The listing builds one solid part. Answer for the finished solid, in the listing's coordinates (mm). Face numbers are marked on the shaded views. A direction names the side the tool comes from. Round coordinates to 2 decimals unless told otherwise and drop trailing zeros. Loops run counter-clockwise (first coordinate to the right, second up) from the corner with the lowest first, then second, coordinate; pieces in that order, holes last. Notation, with made-up numbers: (7, 57.25) -> (31, 57.25) arc R19 ccw to (31, 86.25) -> close; hole circle Ø1 at (-7.5, 46). An arc over 180 degrees is marked (long way). Write each question's results on one line, items separated by ' | '. Start each with the question number.
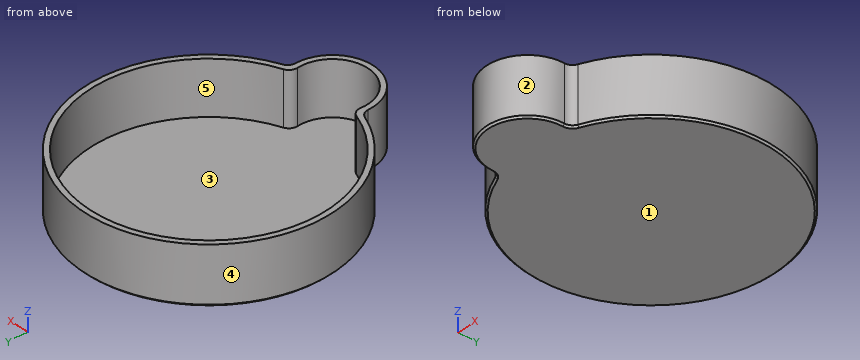
from build123d import *

# Parameters (mm, degrees)
F1_DEPTH = 30
F3_DEPTH = 2
F4_SIZE  = 1


with BuildPart() as f1:
    # F0 (on Top) → F1 (new body)
    with BuildSketch(Plane.XY):
        with BuildLine():
            ThreePointArc((22.997395, -69.653827), (23.832678, -66.810928), (26.130373, -64.94))
            ThreePointArc((26.130373, -64.94), (0, 70), (-26.130373, -64.94))
            ThreePointArc((-26.130373, -64.94), (-23.832678, -66.810928), (-22.997395, -69.653827))
            ThreePointArc((-22.997395, -69.653827), (0, -93), (22.997395, -69.653827))
        make_face()
        with BuildLine():
            ThreePointArc((-23.153211, -62.872321), (0, 67), (23.153211, -62.872321))
            ThreePointArc((23.153211, -62.872321), (20.645274, -64.907579), (19.90485, -68.051429))
            ThreePointArc((19.90485, -68.051429), (0, -90), (-19.90485, -68.051429))
            ThreePointArc((-19.90485, -68.051429), (-20.645274, -64.907579), (-23.153211, -62.872321))
        make_face(mode=Mode.SUBTRACT)
    extrude(amount=F1_DEPTH)

    # F2 (on Top) → F3 (join)
    with BuildSketch(Plane.XY):
        with BuildLine():
            ThreePointArc((22.997395, -69.653827), (23.832678, -66.810928), (26.130373, -64.94))
            ThreePointArc((26.130373, -64.94), (0, 70), (-26.130373, -64.94))
            ThreePointArc((-26.130373, -64.94), (-23.832678, -66.810928), (-22.997395, -69.653827))
            ThreePointArc((-22.997395, -69.653827), (0, -93), (22.997395, -69.653827))
        make_face()
    extrude(amount=-F3_DEPTH)

    # F4
    f4_edges = [f1.edges().sort_by_distance(p)[0] for p in [
        (0, 70, -2),
    ]]
    chamfer(f4_edges, length=F4_SIZE)


solid = f1.part
Item 1: Straight lines are drawn through the part: L1, parallel to X at y = 0, z = 12; L2, parallel to X at y = -70, z = 13.75; L3, parallel to Z at x = 29, y = 21. For each, find the intervals that lie inside material, in ascending order. Write a range as [from, to].
Item 2: Each of these flat-tipped pins is pushed along its axis until it touches: pin 1 Ø10 at (y, z) = (48.5, 25.5) entering from +X; pin 2 Ø6 at (y, z) = (28, 26.5) entering from -X; pin 3 Ø1 at (x, y) = (42.5, 43) entering from +Z. Where does it stop, or does it pass through?
Item 3: The part is cut by section B-B, the plane x = 0. Give the vertices of the cut face in (y, z).
Item 4: For the marked faces 4 and 5, determine the directions among +Z, -Z, +X, -X, +Y, -Y from which every point of the face is accessible in a straight line to the end or side of a thin tool.
Item 5: Determine the mould class of the marked faces 1, 2 and 3 for opening direction X: +X half, -X half, draft (parallel to the pull), parting line (faces both ways), or undercut.
Item 6: The part is cut by section A-A, the plane y = 0. Give the vertices of the cut face in (x, z).
Report:
1) L1: x = [-70, -67], [67, 70] | L2: x = [-23, -20], [20, 23] | L3: z = [-2, 0]
2) pin 1: stops at x = 54.84 | pin 2: stops at x = -65.38 | pin 3: stops at z = 0
3) outline: (-93, -1) -> (-92, -2) -> (69, -2) -> (70, -1) -> (70, 30) -> (67, 30) -> (67, 0) -> (-90, 0) -> (-90, 30) -> (-93, 30) -> close
4) face 4: +Z, -Z | face 5: +Z
5) face 1: draft | face 2: parting line | face 3: undercut
6) outline: (-70, -1) -> (-69, -2) -> (69, -2) -> (70, -1) -> (70, 30) -> (67, 30) -> (67, 0) -> (-67, 0) -> (-67, 30) -> (-70, 30) -> close
